Work out the finished part from the listing and answer in its coordinate system (mm). Face numbers are marked on the shaded views. A direction names the side the tool comes from. Give positions to 0.01 mm unless a question says otherwise; leave off trailing zeros. Loops run counter-clockwise (first coordinate to the right, second up) from the corner with the lowest first, then second, coordinate; pieces in that order, holes last. Notation, with made-up numbers: M -31.5,44.25 L -19.5,44.25 A29 ccw -19.5,82.25 Z; hole C 46,67 d7. An arc over 180 degrees is marked long. Use a Markdown table: item, result.
```python
from build123d import *

# Parameters (mm, degrees)
SKETCH1_R           = 2.5
BOSS_EXTRUDE1_DEPTH = 30


with BuildPart() as part:
    # Sketch1 → Boss-Extrude1 (new body)
    with BuildSketch(Plane(origin=(0, 0, 0), x_dir=(1, 0, 0), z_dir=(0, 1, 0))):
        with Locations(Location((0, 0, 0), (0, 0, 270))):
            Circle(SKETCH1_R)
    extrude(amount=BOSS_EXTRUDE1_DEPTH)

    # Sketch2 → Revolve1 (revolve)
    with BuildSketch(Plane.XY):
        with BuildLine():
            Line((0, 0), (0, -5))
            Line((0, -5), (-5.5, -5))
            ThreePointArc((-5.5, -5), (-6.207106781, -4.707106781), (-6.5, -4))
            Line((-6.5, -4), (-6.5, -1))
            ThreePointArc((-6.5, -1), (-6.207106781, -0.292893219), (-5.5, 0))
            Line((-5.5, 0), (0, 0))
        make_face()
    revolve(axis=Axis((0, 0, 0), (0, -1, 0)))


solid = part.part
```
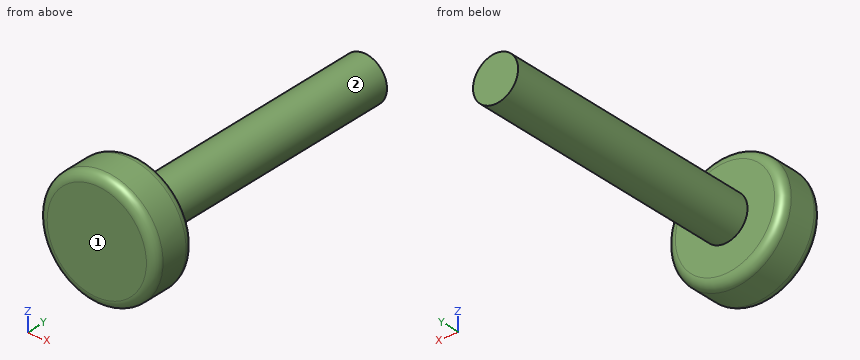
(1) Given P1, Ø1.5, axis at y = 23.5, z = 2, coming from the -X side; P2, Ø4, axis at x = 0, y = 25, coming from the +Z side; P3, Ø6, axis at y = 10.5, z = -1.5, coming from the -X side, each flat-ended and moving along its own axis, determine where each tip first touches the part or whether it passes through.
Entries:
| item | result |
|---|---|
| P1 | stops at x = -2.17 |
| P2 | stops at z = 2.5 |
| P3 | stops at x = -2.5 |
(2) A cutting plane is placed at B-B (x = 0). Write down the section's boundary in (y, z).
Entries:
| item | result |
|---|---|
| outline | M -5,-5.5 A1 ccw -4,-6.5 L -1,-6.5 A1 ccw 0,-5.5 L 0,-2.5 L 30,-2.5 L 30,2.5 L 0,2.5 L 0,5.5 A1 ccw -1,6.5 L -4,6.5 A1 ccw -5,5.5 Z |
(3) A cutting plane is placed at C-C (y = 16). Write down the section's boundary in (x, z).
Entries:
| item | result |
|---|---|
| outline | C 0,0 d5 |
(4) A cutting plane is placed at A-A (z = 0). Write down the section's boundary in (x, y).
Entries:
| item | result |
|---|---|
| outline | M -6.5,-4 A1 ccw -5.5,-5 L 5.5,-5 A1 ccw 6.5,-4 L 6.5,-1 A1 ccw 5.5,0 L 2.5,0 L 2.5,30 L -2.5,30 L -2.5,0 L -5.5,0 A1 ccw -6.5,-1 Z |
(5) Consider probe 1 along Y at (x, z) = (-5, -0.5); probe 2 along Z at (x, y) = (-0.25, -1.5); probe 3 along X at (y, z) = (17.5, 2). Determine where each line is inside the solid, lowest interval first. Write a range as [from, to].
Entries:
| item | result |
|---|---|
| probe 1 | y = [-5, 0] |
| probe 2 | z = [-6.5, 6.5] |
| probe 3 | x = [-1.5, 1.5] |
(6) Which of the six approach directions +Z, -Z, +X, -X, +Y, -Y give full straight-line access (tool end or side, diameter ignored) to the marked faces 1 and 2?
Entries:
| item | result |
|---|---|
| face 1 | +Z, -Z, +X, -X, -Y |
| face 2 | +Y |
